Autodesk Inventor part; units mm, degrees
ref_plane "YZ Plane" through (0, 0, 0) normal (1, 0, 0) x (0, 1, 0)
ref_plane "XZ Plane" through (0, 0, 0) normal (0, 1, 0) x (-1, 0, 0)
ref_plane "XY Plane" through (0, 0, 0) normal (0, 0, 1) x (1, 0, 0)
sketch "Sketch1" plane through (0, 0, 0) normal (0, 0, 1) x (1, 0, 0)
  line L0 (0, 0) -> (25.4, 0)
  line L1 (25.4, 0) -> (25.4, 50.8)
  line L2 (25.4, 50.8) -> (0, 50.8)
  line L3 (0, 50.8) -> (0, 0)
  dimension "d0" = 25.4
  dimension "d1" = 50.8
extrude "Extrusion1" add sketch "Sketch1" along normal blind 152.4
shell "Shell1" thickness 3.175 removed faces 2 at (8.4667, 33.8667, 0) at (8.4667, 33.8667, 152.4)
sketch "Sketch4" plane through (25.4, 0, 0) normal (1, 0, 0) x (0, 0, -1)
  line L0 (-152.4, 50.8) -> (-152.4, 0)
  line L1 (0, 0) -> (-152.4, 0)
  line L2 (0, 50.8) -> (-152.4, 50.8)
  line L3 (-152.4, 44.45) -> (-114.3, 44.45)
  line L4 (-114.3, 44.45) -> (-114.3, 6.35)
  line L5 (-114.3, 6.35) -> (-152.4, 6.35)
  line L6 (-152.4, 6.35) -> (-152.4, 44.45)
  dimension "d15" = 6.35
  dimension "d16" = 6.35
  dimension "d17" = 38.1
extrude "Extrusion4" cut sketch "Sketch4" against normal through all
sketch "Sketch5" plane through (0, 50.8, 0) normal (0, 1, 0) x (1, 0, 0)
  line L0 (0, -152.4) -> (25.4, -152.4)
  line L1 (25.4, 0) -> (25.4, -152.4)
  circle A0 centre (12.7, -139.7) radius 3.9688
  dimension "d20" = 7.9375
  dimension "d21" = 12.7
  dimension "d22" = 12.7
extrude "Extrusion5" cut sketch "Sketch5" against normal through all
properties part number "Frame_LowerRollerMount" material "Aluminum-6061"
Build history of the part. All positions in model axes, mm. A direction names the side the tool comes from. Give positions to 0.01 mm unless a question says otherwise; leave off trailing zeros. Order: outer loops, then holes, each group sorted by start corner. A loop starts at its lowest first (then second) coordinate and runs counter-clockwise, first axis right, second up. Notation, with made-up numbers: M -34.75,-3.75 L -7.75,-3.75 A16 ccw -7.75,27.25 Z; hole C 34.25,30 d10. An arc over 180 degrees is marked long. Use one line per item in the form item = value.
1) Two-plate mould, pull along Z, no slides. Class faces 4 (the face through (13, 2, 152.4)), 5 (the face through (11.84, 49.235, 143.574)), 6 (the face through (25.4, 25, 58)): released by +Z, released by -Z, zero draft, split by the parting line, or undercut.
Calculated:
face_4 = released by +Z
face_5 = undercut
face_6 = zero draft
2) Saw through at C-C (z = 117.5). Give the cut face in (x, y) (3 decimals).
Calculated:
outline = M 0,0 L 25.4,0 L 25.4,6.35 L 22.225,6.35 L 22.225,3.175 L 3.175,3.175 L 3.175,6.35 L 0,6.35 Z; M 0,44.45 L 3.175,44.45 L 3.175,47.625 L 22.225,47.625 L 22.225,44.45 L 25.4,44.45 L 25.4,50.8 L 0,50.8 Z
3) Probe probe 1 along Y at (x, z) = (6.5, 7) (3 decimals); probe 2 along Z at (x, y) = (12.7, 2.05); probe 3 along X at (y, z) = (20, 86) (3 decimals). List the from-to ranges inside material, lowest first.
Calculated:
probe_1 = 0 to 3.175, 47.625 to 50.8
probe_2 = 0 to 135.73, 143.67 to 152.4
probe_3 = 0 to 3.175, 22.225 to 25.4
4) Saw through at D-D (z = 139.7). Give the cut face in (x, y) (3 decimals), plus the area to 3 significant figures.
Calculated:
outline = M 0,0 L 8.731,0 L 8.731,3.175 L 3.175,3.175 L 3.175,6.35 L 0,6.35 Z; M 0,44.45 L 3.175,44.45 L 3.175,47.625 L 8.731,47.625 L 8.731,50.8 L 0,50.8 Z; M 16.669,0 L 25.4,0 L 25.4,6.35 L 22.225,6.35 L 22.225,3.175 L 16.669,3.175 Z; M 16.669,47.625 L 22.225,47.625 L 22.225,44.45 L 25.4,44.45 L 25.4,50.8 L 16.669,50.8 Z
area = 151 mm2
5) Tool access for faces 1 (the face through (11.84, 1.61, 143.574)), 2 (the face through (13, 3.175, 75)), 3 (the face through (2, 26, 114.3)): list every direction of +Z, -Z, +X, -X, +Y, -Y with a clear straight run to the whole face (end or side of a thin tool).
Calculated:
face_1 = +Y, -Y
face_2 = +Z, -Z
face_3 = +Z, +X, -X
6) Saw through at B-B (x = 12.7). Give the cut face in (y, z) (3 decimals).
Calculated:
outline = M 0,0 L 3.175,0 L 3.175,135.731 L 0,135.731 Z; M 0,143.669 L 3.175,143.669 L 3.175,152.4 L 0,152.4 Z; M 47.625,0 L 50.8,0 L 50.8,135.731 L 47.625,135.731 Z; M 47.625,143.669 L 50.8,143.669 L 50.8,152.4 L 47.625,152.4 Z
7) Drop flat-ended pins along their axis: pin 1 (9.5 mm diameter, centred on x = 12, z = 95, fed in from -Y); pin 2 (2.5 mm diameter, centred on x = 24, y = 20.5, fed in from +Z); pin 3 (10 mm diameter, centred on x = 14.5, y = 37.5, fed in from -Z). Give the stop position or say it passes through.
Calculated:
pin_1 = 0
pin_2 = 114.3
pin_3 = through
8) Saw through at A-A (y = 8). Give the cut face in (x, z) (3 decimals), plus the area to 3 significant figures.
Calculated:
outline = M 0,0 L 3.175,0 L 3.175,114.3 L 0,114.3 Z; M 22.225,0 L 25.4,0 L 25.4,114.3 L 22.225,114.3 Z
area = 726 mm2
